Work out the finished part from the listing and answer in its coordinate system (mm). A direction names the side the tool comes from. Coordinates: 2 decimals unless noted, no trailing zeros. Write each loop counter-clockwise with the first axis right and the second up, starting at its lowest first coordinate (ties: lowest second). Pieces come first, ordered by that corner, then holes. Notation, with made-up numbers: M 41,-31 L 98,-31 A17 cw 98,-13 Z; hole C 29.5,21 d2. An arc over 180 degrees is marked long. Answer as CSV lines item,"result". Start each with the question number.
(1) The mould has two halves that part along X. Classify faces 1 (the flat face through (0.85, 43.4, 0)), 2 (the cylindrical face through (-0.867, 33.153, -3.905)), 3 (the flat face through (0, 23.5, -2.2)): released by +X, released by -X, zero draft, split by the parting line, or undercut.
(2) Flat-ended cylindrical pins translate along their axes: P1, Ø0.5, axis at x = 0, z = -1.5, coming from the +Y side; P2, Ø1, axis at x = -2, y = 13.5, coming from the +Z side; P3, Ø4, axis at x = 1, y = 6, coming from the +Z side. Find the tip coordinate at first contact, or state that the pin passes through.
(3) A cutting plane is placed at A-A on y = 15. Give the vertices of the cut face in (x, z), then the cut area to 3 significant figures.
(4) A cutting plane is placed at B-B on y = 35.5. Give the vertices of the cut face in (x, z).
(5) Find the intervals of material crossed by L1, parallel to X at y = 26.5, z = 0.25; L2, parallel to Y at x = 0, z = -2.75; L3, parallel to Z at x = 1.75, y = 33, in increasing order. Write a range as [from, to].
(6) For faces 4 (the flat face through (-0.85, 43.4, 0)), 5 (the cylindrical face through (0, 13, -2)), determine the directions among +Z, -Z, +X, -X, +Y, -Y from which every point of the face is accessible in a straight line to the end or side of a thin tool.
from build123d import *

# Parameters (mm, degrees)
DOME_1_FACE_RADIUS       = 4
DOME_1_HEIGHT            = 2
SKETCH_3_W               = 1.7
SKETCH_3_H               = 10
CUT_EXTRUDE_1_DEPTH      = 5
CUT_EXTRUDE_1_DEPTH_BACK = 5
CHAMFER_1_SIZE           = 0.5545


with BuildPart() as part:
    # Sketch 2 → Revolve 1 (revolve)
    with BuildSketch(Plane.XY):
        Polygon((0, 0), (2, 1.5), (2, 23.5), (4, 23.5), (4, 42), (0, 42), align=None)
    revolve(axis=Axis((0, 42, 0), (0, -1, 0)))

    # Dome 1: a dome of height H over a round flat face of radius A is a cap of a sphere of radius (A * A + H * H) / (2 * H)
    dome_1_r = (DOME_1_FACE_RADIUS * DOME_1_FACE_RADIUS + DOME_1_HEIGHT * DOME_1_HEIGHT) / (2 * DOME_1_HEIGHT)
    dome_1_base = Plane((0, 42, 0), z_dir=(0, 1, 0))
    with Locations(dome_1_base.offset(DOME_1_HEIGHT - dome_1_r)):
        dome_1_ball = Sphere(dome_1_r, mode=Mode.PRIVATE)
    add(split(dome_1_ball, bisect_by=dome_1_base, keep=Keep.TOP, mode=Mode.PRIVATE))

    # Sketch 3 → Cut-Extrude 1 (cut, two sides)
    with BuildSketch(Plane.XY) as cut_extrude_1_sk:
        with Locations((0, 48)):
            Rectangle(SKETCH_3_W, SKETCH_3_H)
    extrude(amount=CUT_EXTRUDE_1_DEPTH, mode=Mode.SUBTRACT)
    extrude(cut_extrude_1_sk.sketch, amount=-CUT_EXTRUDE_1_DEPTH_BACK, mode=Mode.SUBTRACT)

    # Chamfer 1
    chamfer_1_edges = [part.edges().sort_by_distance(p)[0] for p in [
        (-4, 23.5, 0),
    ]]
    chamfer(chamfer_1_edges, length=CHAMFER_1_SIZE)


solid = part.part
Here are the results:
1,face 1,"undercut"
1,face 2,"split by the parting line"
1,face 3,"zero draft"
2,P1,"stops at y = 43"
2,P2,"stops at z = 1.32"
2,P3,"stops at z = 2"
3,outline,"C 0,0 d4"
3,area,"12.6 mm^2"
4,outline,"C 0,0 d8"
5,L1,"x = [-3.99, 3.99]"
5,L2,"y = [23.5, 43]"
5,L3,"z = [-3.6, 3.6]"
6,face 4,"+Z, -Z, +Y"
6,face 5,"-Y"
